Input: part model. Units: mm. Frame: model coordinates. Give positions to 0.01 mm unless a question says otherwise; leave off trailing zeros. Loops run counter-clockwise (first coordinate to the right, second up) from the corner with the lowest first, then second, coordinate; pieces in that order, holes last. Notation, with made-up numbers: M -9.75,64.5 L 42.25,64.5 A21 ccw 42.25,102.5 Z; hole C -1,-34 d5. An arc over 180 degrees is marked long. Return JSON: item names as keys, results as strings. Group by question number.
```python
from build123d import *

# Parameters (mm, degrees)
SKETCH1_R           = 2
SKETCH1_R_2         = 3.5
BOSS_EXTRUDE1_DEPTH = 320
FILLET1_R           = 0.2
FILLET2_R           = 0.2


with BuildPart() as part:
    # Sketch1 → Boss-Extrude1 (new body)
    with BuildSketch(Plane.XY):
        with BuildLine():
            Line((-5, 3), (-5, -3))
            Line((-5, -3), (-7, -3))
            Line((-7, -3), (-7, -5))
            Line((-7, -5), (-13.5, -5))
            Line((-13.5, -5), (-13.5, -3))
            Line((-13.5, -3), (-15, -3))
            Line((-15, -3), (-15, -27))
            Line((-15, -27), (-13.5, -27))
            Line((-13.5, -27), (-13.5, -25))
            Line((-13.5, -25), (-7, -25))
            Line((-7, -25), (-7, -27))
            Line((-7, -27), (-5, -27))
            Line((-5, -27), (-5, -33))
            Line((-5, -33), (-7, -33))
            Line((-7, -33), (-7, -35))
            Line((-7, -35), (-13.5, -35))
            Line((-13.5, -35), (-13.5, -33))
            Line((-13.5, -33), (-15, -33))
            Line((-15, -33), (-15, -44))
            ThreePointArc((-15, -44), (-14.707106781, -44.707106781), (-14, -45))
            Line((-14, -45), (-3, -45))
            Line((-3, -45), (-3, -43.5))
            Line((-3, -43.5), (-5, -43.5))
            Line((-5, -43.5), (-5, -38.87437693))
            Line((-5, -38.87437693), (-3, -38.87437693))
            Line((-3, -38.87437693), (-3, -36.87437693))
            Line((-3, -36.87437693), (3, -36.87437693))
            Line((3, -36.87437693), (3, -38.87437693))
            Line((3, -38.87437693), (5, -38.87437693))
            Line((5, -38.87437693), (5, -43.5))
            Line((5, -43.5), (3, -43.5))
            Line((3, -43.5), (3, -45))
            Line((3, -45), (27, -45))
            Line((27, -45), (27, -43.5))
            Line((27, -43.5), (25, -43.5))
            Line((25, -43.5), (25, -38.87437693))
            Line((25, -38.87437693), (27, -38.87437693))
            Line((27, -38.87437693), (27, -36.87437693))
            Line((27, -36.87437693), (33, -36.87437693))
            Line((33, -36.87437693), (33, -38.87437693))
            Line((33, -38.87437693), (35, -38.87437693))
            Line((35, -38.87437693), (35, -43.5))
            Line((35, -43.5), (33, -43.5))
            Line((33, -43.5), (33, -45))
            Line((33, -45), (44, -45))
            ThreePointArc((44, -45), (44.707106781, -44.707106781), (45, -44))
            Line((45, -44), (45, -33))
            Line((45, -33), (43.5, -33))
            Line((43.5, -33), (43.5, -35))
            Line((43.5, -35), (37, -35))
            Line((37, -35), (37, -33))
            Line((37, -33), (35, -33))
            Line((35, -33), (35, -27))
            Line((35, -27), (37, -27))
            Line((37, -27), (37, -25))
            Line((37, -25), (43.5, -25))
            Line((43.5, -25), (43.5, -27))
            Line((43.5, -27), (45, -27))
            Line((45, -27), (45, -3))
            Line((45, -3), (43.5, -3))
            Line((43.5, -3), (43.5, -5))
            Line((43.5, -5), (37, -5))
            Line((37, -5), (37, -3))
            Line((37, -3), (35, -3))
            Line((35, -3), (35, 3))
            Line((35, 3), (37, 3))
            Line((37, 3), (37, 5))
            Line((37, 5), (43.5, 5))
            Line((43.5, 5), (43.5, 3))
            Line((43.5, 3), (45, 3))
            Line((45, 3), (45, 14))
            ThreePointArc((45, 14), (44.707106781, 14.707106781), (44, 15))
            Line((44, 15), (33, 15))
            Line((33, 15), (33, 13.5))
            Line((33, 13.5), (35, 13.5))
            Line((35, 13.5), (35, 8.87437693))
            Line((35, 8.87437693), (33, 8.87437693))
            Line((33, 8.87437693), (33, 6.87437693))
            Line((33, 6.87437693), (27, 6.87437693))
            Line((27, 6.87437693), (27, 8.87437693))
            Line((27, 8.87437693), (25, 8.87437693))
            Line((25, 8.87437693), (25, 13.5))
            Line((25, 13.5), (27, 13.5))
            Line((27, 13.5), (27, 15))
            Line((27, 15), (3, 15))
            Line((3, 15), (3, 13.5))
            Line((3, 13.5), (5, 13.5))
            Line((5, 13.5), (5, 8.87437693))
            Line((5, 8.87437693), (3, 8.87437693))
            Line((3, 8.87437693), (3, 6.87437693))
            Line((3, 6.87437693), (-3, 6.87437693))
            Line((-3, 6.87437693), (-3, 8.87437693))
            Line((-3, 8.87437693), (-5, 8.87437693))
            Line((-5, 8.87437693), (-5, 13.5))
            Line((-5, 13.5), (-3, 13.5))
            Line((-3, 13.5), (-3, 15))
            Line((-3, 15), (-14, 15))
            ThreePointArc((-14, 15), (-14.707106781, 14.707106781), (-15, 14))
            Line((-15, 14), (-15, 3))
            Line((-15, 3), (-13.5, 3))
            Line((-13.5, 3), (-13.5, 5))
            Line((-13.5, 5), (-7, 5))
            Line((-7, 5), (-7, 3))
            Line((-7, 3), (-5, 3))
        make_face()
        Circle(SKETCH1_R, mode=Mode.SUBTRACT)
        with Locations((-10.606601718, 10.606601718)):
            Circle(SKETCH1_R_2, mode=Mode.SUBTRACT)
        with Locations((-10.606601718, -40.606601718)):
            Circle(SKETCH1_R_2, mode=Mode.SUBTRACT)
        with Locations((0, -30)):
            Circle(SKETCH1_R, mode=Mode.SUBTRACT)
        with Locations((40.606601718, 10.606601718)):
            Circle(SKETCH1_R_2, mode=Mode.SUBTRACT)
        with Locations((30, 0)):
            Circle(SKETCH1_R, mode=Mode.SUBTRACT)
        with Locations((30, -30)):
            Circle(SKETCH1_R, mode=Mode.SUBTRACT)
        with Locations((40.606601718, -40.606601718)):
            Circle(SKETCH1_R_2, mode=Mode.SUBTRACT)
        with BuildLine():
            Line((7, 6), (4, 3))
            ThreePointArc((4, 3), (3.276008707, -3.777269775), (-3.535533906, -3.535533906))
            Line((-3.535533906, -3.535533906), (-7, -7))
            Line((-7, -7), (-11, -7))
            ThreePointArc((-11, -7), (-11.707106781, -7.292893219), (-12, -8))
            Line((-12, -8), (-12, -22))
            ThreePointArc((-12, -22), (-11.707106781, -22.707106781), (-11, -23))
            Line((-11, -23), (-7, -23))
            Line((-7, -23), (-3.535533906, -26.464466094))
            ThreePointArc((-3.535533906, -26.464466094), (3.276008707, -26.222730225), (4, -33))
            Line((4, -33), (7, -36))
            Line((7, -36), (7, -41))
            ThreePointArc((7, -41), (7.292893219, -41.707106781), (8, -42))
            Line((8, -42), (22, -42))
            ThreePointArc((22, -42), (22.707106781, -41.707106781), (23, -41))
            Line((23, -41), (23, -36))
            Line((23, -36), (26, -33))
            ThreePointArc((26, -33), (26.723991293, -26.222730225), (33.535533906, -26.464466094))
            Line((33.535533906, -26.464466094), (37, -23))
            Line((37, -23), (41, -23))
            ThreePointArc((41, -23), (41.707106781, -22.707106781), (42, -22))
            Line((42, -22), (42, -8))
            ThreePointArc((42, -8), (41.707106781, -7.292893219), (41, -7))
            Line((41, -7), (37, -7))
            Line((37, -7), (33.535533906, -3.535533906))
            ThreePointArc((33.535533906, -3.535533906), (26.723991293, -3.777269775), (26, 3))
            Line((26, 3), (23, 6))
            Line((23, 6), (23, 11))
            ThreePointArc((23, 11), (22.707106781, 11.707106781), (22, 12))
            Line((22, 12), (8, 12))
            ThreePointArc((8, 12), (7.292893219, 11.707106781), (7, 11))
            Line((7, 11), (7, 6))
        make_face(mode=Mode.SUBTRACT)
    extrude(amount=BOSS_EXTRUDE1_DEPTH)

    # Fillet1
    fillet1_edges = [part.edges().sort_by_distance(p)[0] for p in [
        (-15, 3, 160),
        (-3, 15, 160),
        (3, 15, 160),
        (27, 15, 160),
        (33, 15, 160),
        (45, 3, 160),
        (45, -3, 160),
        (45, -27, 160),
        (45, -33, 160),
        (33, -45, 160),
        (27, -45, 160),
        (3, -45, 160),
        (-3, -45, 160),
        (-15, -33, 160),
        (-15, -27, 160),
        (-15, -3, 160),
    ]]
    fillet(fillet1_edges, radius=FILLET1_R)

    # Fillet2
    fillet2_edges = [part.edges().sort_by_distance(p)[0] for p in [
        (-13.5, 3, 160),
        (-3, 13.5, 160),
        (3, 13.5, 160),
        (27, 13.5, 160),
        (33, 13.5, 160),
        (43.5, 3, 160),
        (43.5, -3, 160),
        (43.5, -27, 160),
        (43.5, -33, 160),
        (33, -43.5, 160),
        (27, -43.5, 160),
        (3, -43.5, 160),
        (-3, -43.5, 160),
        (-13.5, -33, 160),
        (-13.5, -27, 160),
        (-13.5, -3, 160),
    ]]
    fillet(fillet2_edges, radius=FILLET2_R)


solid = part.part
```
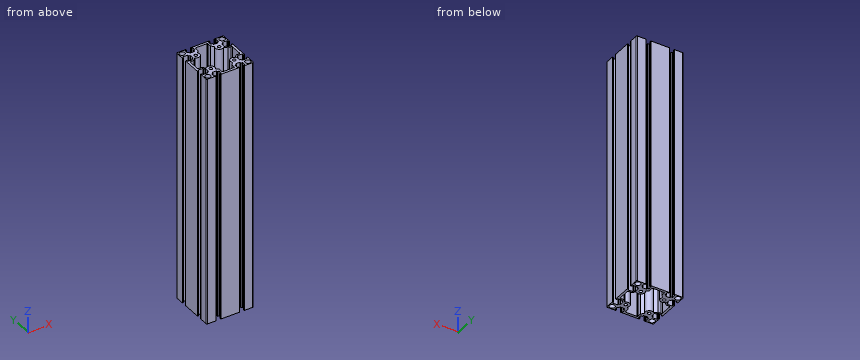
Item 1: Section A-A, the plane x = 14. Return loops of the section in (y, z).
Item 2: Material intervals for line 1 (Y direction, x = 0, z = 133); line 2 (Y direction, x = 40.5, z = 44); line 3 (Y direction, x = 13, z = 205), sorted ascending. Write a range as from..to.
Item 3: Section C-C, the plane z = 171.5. Give the number of separate pieces and of enclosed holes in the cut face, then the cut area to 3 significant figures.
Item 4: Section B-B, the plane y = -13.5. Return loops of the section in (x, z).
Item 5: First-contact query: pin 1 Ø3 at (x, z) = (-0.5, 172.5) entering from -Y. Flat tip, straight axial feed; report the tip coordinate or a pass-through.
Answer below:
{
 "1": {"outline": "M -45,0 L -42,0 L -42,320 L -45,320 Z; M 12,0 L 15,0 L 15,320 L 12,320 Z"},
 "2": {"line 1": "-36.87..-32, -28..-25, -5..-2, 2..6.87", "line 2": "-45..-44.1, -37.11..-35, -25..-23, -7..-5, 5..7.11, 14.1..15", "line 3": "-45..-42, 12..15"},
 "3": {"separate pieces": "1", "enclosed holes": "9", "area": "1,090 mm^2"},
 "4": {"outline": "M -15,0 L -12,0 L -12,320 L -15,320 Z; M 42,0 L 45,0 L 45,320 L 42,320 Z"},
 "5": {"pin 1": "y = -36.87"}
}
